from build123d import *

# Parameters (mm, degrees)
CUT_EXTRUDE2_DEPTH = 3.175
CUT_EXTRUDE3_DEPTH = 3.175


with BuildPart() as part:
    # Sketch1 → Revolve1 (revolve)
    with BuildSketch(Plane.XY):
        with BuildLine():
            Line((6.35, 154.305), (14.605, 154.305))
            Line((14.605, 154.305), (14.605, 145.923))
            Line((14.605, 145.923), (30.329807741, 143.593398853))
            ThreePointArc((30.329807741, 143.593398853), (31.517982802, 143.084998901), (32.302189527, 142.057745136))
            Line((32.302189527, 142.057745136), (34.925, 135.763))
            Line((34.925, 135.763), (34.925, 126.238))
            Line((34.925, 126.238), (32.385, 124.968))
            Line((32.385, 124.968), (32.385, 13.12493032))
            ThreePointArc((32.385, 13.12493032), (31.763853046, 11.460717897), (30.204210245, 10.610458606))
            Line((30.204210245, 10.610458606), (14.605, 8.382))
            Line((14.605, 8.382), (14.605, 0))
            Line((14.605, 0), (6.35, 0))
            Line((6.35, 0), (6.35, 10.409948615))
            Line((6.35, 10.409948615), (29.21, 13.6756629))
            Line((29.21, 13.6756629), (29.21, 140.549643155))
            Line((29.21, 140.549643155), (6.35, 143.936309822))
            Line((6.35, 143.936309822), (6.35, 154.305))
        make_face()
    revolve(axis=Axis((0, 0, 0), (0, 1, 0)))

    # Sketch2 → Cut-Extrude2 (cut)
    with BuildSketch(Plane.XZ):
        with BuildLine():
            Line((1.5875, -12.920338618), (1.5875, -9.391776656))
            ThreePointArc((1.5875, -9.391776656), (6.735192091, -6.735192091), (9.391776656, -1.5875))
            Line((9.391776656, -1.5875), (12.920338618, -1.5875))
            ThreePointArc((12.920338618, -1.5875), (9.204762524, -9.204762524), (1.5875, -12.920338618))
        make_face()
        with BuildLine():
            Line((-1.5875, -12.920338618), (-1.5875, -9.391776656))
            ThreePointArc((-1.5875, -9.391776656), (-6.735192091, -6.735192091), (-9.391776656, -1.5875))
            Line((-9.391776656, -1.5875), (-12.920338618, -1.5875))
            ThreePointArc((-12.920338618, -1.5875), (-9.204762524, -9.204762524), (-1.5875, -12.920338618))
        make_face()
        with BuildLine():
            Line((-12.920338618, 1.5875), (-9.391776656, 1.5875))
            ThreePointArc((-9.391776656, 1.5875), (-6.735192091, 6.735192091), (-1.5875, 9.391776656))
            Line((-1.5875, 9.391776656), (-1.5875, 12.920338618))
            ThreePointArc((-1.5875, 12.920338618), (-9.204762524, 9.204762524), (-12.920338618, 1.5875))
        make_face()
        with BuildLine():
            Line((1.5875, 12.920338618), (1.5875, 9.391776656))
            ThreePointArc((1.5875, 9.391776656), (6.735192091, 6.735192091), (9.391776656, 1.5875))
            Line((9.391776656, 1.5875), (12.920338618, 1.5875))
            ThreePointArc((12.920338618, 1.5875), (9.204762524, 9.204762524), (1.5875, 12.920338618))
        make_face()
    extrude(amount=-CUT_EXTRUDE2_DEPTH, mode=Mode.SUBTRACT)

    # Sketch3 → Cut-Extrude3 (cut)
    with BuildSketch(Plane(origin=(0, 154.305, 0), x_dir=(-1, 0, 0), z_dir=(0, 1, 0))):
        with BuildLine():
            Line((1.5875, -12.920338618), (1.5875, -9.391776656))
            ThreePointArc((1.5875, -9.391776656), (6.735192091, -6.735192091), (9.391776656, -1.5875))
            Line((9.391776656, -1.5875), (12.920338618, -1.5875))
            ThreePointArc((12.920338618, -1.5875), (9.204762524, -9.204762524), (1.5875, -12.920338618))
        make_face()
        with BuildLine():
            Line((-1.5875, -12.920338618), (-1.5875, -9.391776656))
            ThreePointArc((-1.5875, -9.391776656), (-6.735192091, -6.735192091), (-9.391776656, -1.5875))
            Line((-9.391776656, -1.5875), (-12.920338618, -1.5875))
            ThreePointArc((-12.920338618, -1.5875), (-9.204762524, -9.204762524), (-1.5875, -12.920338618))
        make_face()
        with BuildLine():
            Line((-12.920338618, 1.5875), (-9.391776656, 1.5875))
            ThreePointArc((-9.391776656, 1.5875), (-6.735192091, 6.735192091), (-1.5875, 9.391776656))
            Line((-1.5875, 9.391776656), (-1.5875, 12.920338618))
            ThreePointArc((-1.5875, 12.920338618), (-9.204762524, 9.204762524), (-12.920338618, 1.5875))
        make_face()
        with BuildLine():
            Line((1.5875, 12.920338618), (1.5875, 9.391776656))
            ThreePointArc((1.5875, 9.391776656), (6.735192091, 6.735192091), (9.391776656, 1.5875))
            Line((9.391776656, 1.5875), (12.920338618, 1.5875))
            ThreePointArc((12.920338618, 1.5875), (9.204762524, 9.204762524), (1.5875, 12.920338618))
        make_face()
    extrude(amount=-CUT_EXTRUDE3_DEPTH, mode=Mode.SUBTRACT)


solid = part.part
For this review, take the finished solid that the model builds, in its own axes (mm). A direction names the side the tool comes from. Round coordinates to 2 decimals unless told otherwise and drop trailing zeros. Write each loop counter-clockwise with the first axis right and the second up, starting at its lowest first coordinate (ties: lowest second). Pieces come first, ordered by that corner, then holes. Notation, with made-up numbers: (-21.5, 39) -> (4.5, 39) arc R29 ccw to (4.5, 69) -> close; hole circle Ø1 at (-40, -14). An arc over 180 degrees is marked (long way). Put each result on its own line as item: value.
Q1. Machinability: for faces 1 (the cylindrical face through (6.79, 152.74, 6.68)), 2 (the flat face through (7, 3.175, -7)), 3 (the cylindrical face through (-1.38, 149.19, 6.2)), which of the approach directions +Z, -Z, +X, -X, +Y, -Y give a long, thin tool a straight path to every point of the face, cutting with its end or side? Answer none if there is none.
Determined:
face 1: +Y
face 2: -Y
face 3: +Y, -Y
Q2. To check wall thickness, follow L1, parallel to X at y = 151.5, z = 0 (3 decimals); L2, parallel to X at y = 65.5, z = 0 (3 decimals). State the ranges of each line that lie inside material, in increasing order. Write a range as [from, to].
Determined:
L1: x = [-14.605, -6.35], [6.35, 14.605]
L2: x = [-32.385, -29.21], [29.21, 32.385]
Q3. Clearance check with flat-ended pins moving along their axes: pin 1 Ø1 at (x, y) = (20.5, 39) entering from +Z; pin 2 Ø2 at (y, z) = (99, -19) entering from +X; pin 3 Ø3.5 at (y, z) = (1, -11) entering from -X; pin 4 Ø5.5 at (x, z) = (-5, -10) entering from -Y. State where each tip first meets the part, or that it passes through.
Determined:
pin 1: stops at z = 25.47
pin 2: stops at x = 26.92
pin 3: stops at x = -11.3
pin 4: stops at y = 0
Q4. Consider section C-C on y = 62. State the section outline as (x, z) points (3 decimals), and give its area (3 significant figures).
Determined:
outline: circle Ø64.77 at (0, 0); hole circle Ø58.42 at (0, 0)
area: 614 mm^2
